Verification items for the finished model (mm, model axes). Coordinates: 2 decimals unless noted, no trailing zeros. Write each loop counter-clockwise with the first axis right and the second up, starting at its lowest first coordinate (ties: lowest second). Pieces come first, ordered by that corner, then holes. Notation, with made-up numbers: (-32.5, 65) - (13.5, 65) arc R21 ccw to (13.5, 86) - close; hole circle Ø6 at (38.25, 50). An arc over 180 degrees is marked (long way). Use one line per item in the form item = value. Start each with the question number.
(1) Gauge pin test, flat ends, axial feed: pin 1 Ø1 at (x, z) = (-4, -115) entering from -Y; pin 2 Ø5 at (y, z) = (-5, -49.5) entering from -X; pin 3 Ø6 at (y, z) = (-6, 46) entering from +X. Record the tip position at first contact, or that the pin passes through.
(2) Sectioned sample at B-B (y = 0). Record the cut outline in (x, z), and give its area (4 significant figures).
(3) Mould release check, pull along Y, two halves, no side actions. Record for faces 1 (the cylindrical face through (-1.713, -7.712, 2.275)), 2 (the flat face through (2, 6, 162.5)), 3 (the cylindrical face through (-1.301, -5.857, 2.275)): released by +Y, released by -Y, zero draft, split by the parting line, or undercut.
(4) Material ranges on line 1 (Z direction, x = 3, y = 5.75); line 2 (Y direction, x = 0, z = 89); line 3 (X direction, y = 2.75, z = -132.5), recorded low to high. Write a range as [from, to].
(5) Sectioned sample at C-C (z = -43.5). Record the cut outline in (x, y), and give its area (3 significant figures).
(6) Sectioned sample at A-A (x = 0). Record the cut outline in (y, z).
from build123d import *

# Parameters (mm, degrees)
CROQUIS1_R                 = 7.9
SALIENTE_EXTRUIR1_DEPTH    = 162.5
CROQUIS3_R                 = 6
CORTAR_EXTRUIR1_DEPTH      = 326.191974071
CORTAR_EXTRUIR2_REACH      = 164.884
CORTAR_EXTRUIR2_END_RADIUS = 7.9
CROQUIS4_W                 = 10
CROQUIS4_H                 = 10
CORTAR_EXTRUIR3_REACH      = 164.884
CORTAR_EXTRUIR3_END_RADIUS = 7.9
CROQUIS5_W                 = 9.290487028
CROQUIS5_H                 = 10


with BuildPart() as part:
    # Croquis1 → Saliente-Extruir1 (new, symmetric)
    with BuildSketch(Plane.XY):
        Circle(CROQUIS1_R)
    extrude(amount=SALIENTE_EXTRUIR1_DEPTH, both=True)

    # Croquis3 → Cortar-Extruir1 (cut, through all)
    with BuildSketch(Plane.XY.offset(162.5)):
        Circle(CROQUIS3_R)
    extrude(amount=-CORTAR_EXTRUIR1_DEPTH, mode=Mode.SUBTRACT)

    # Cortar-Extruir2: up to this cylinder (the profile starts inside it)
    cortar_extruir2_end = Plane(origin=(0, 0, 82.5), z_dir=(0, 0, -1)) * Cylinder(CORTAR_EXTRUIR2_END_RADIUS, 346.568, mode=Mode.PRIVATE)
    # Croquis4 → Cortar-Extruir2 (cut, up to the surface)
    with BuildSketch(Plane(origin=(0, 0, 0), x_dir=(1, 0, 0), z_dir=(0, 1, 0)), mode=Mode.PRIVATE) as cortar_extruir2_sk1:
        with Locations((0, -82.5)):
            Rectangle(CROQUIS4_W, CROQUIS4_H)
    cortar_extruir2_tool1 = extrude(cortar_extruir2_sk1.sketch, amount=CORTAR_EXTRUIR2_REACH, mode=Mode.PRIVATE) & cortar_extruir2_end
    add(cortar_extruir2_tool1.solids().sort_by_distance((0, 0, 82.5))[0], mode=Mode.SUBTRACT)

    # Cortar-Extruir3: up to this cylinder (the profile starts inside it)
    cortar_extruir3_end = Plane(origin=(0, 0, -67.5), z_dir=(0, 0, -1)) * Cylinder(CORTAR_EXTRUIR3_END_RADIUS, 346.568, mode=Mode.PRIVATE)
    # Croquis5 → Cortar-Extruir3 (cut, up to the surface)
    with BuildSketch(Plane(origin=(0, 0, 0), x_dir=(1, 0, 0), z_dir=(0, 1, 0)), mode=Mode.PRIVATE) as cortar_extruir3_sk1:
        with Locations((0, 67.5)):
            Rectangle(CROQUIS5_W, CROQUIS5_H)
    cortar_extruir3_tool1 = extrude(cortar_extruir3_sk1.sketch, amount=CORTAR_EXTRUIR3_REACH, mode=Mode.PRIVATE) & cortar_extruir3_end
    add(cortar_extruir3_tool1.solids().sort_by_distance((0, 0, -67.5))[0], mode=Mode.SUBTRACT)


solid = part.part
Answers below:
q1.pin_1 = -7.08
q1.pin_2 = -7.49
q1.pin_3 = 7.31
q2.outline = (-7.9, -162.5) - (-6, -162.5) - (-6, 162.5) - (-7.9, 162.5) - close; (6, -162.5) - (7.9, -162.5) - (7.9, 162.5) - (6, 162.5) - close
q2.area = 1,235 mm2
q3.face_1 = split by the parting line
q3.face_2 = zero draft
q3.face_3 = undercut
q4.line_1 = [-162.5, -72.5], [-62.5, 77.5], [87.5, 162.5]
q4.line_2 = [-7.9, -6], [6, 7.9]
q4.line_3 = [-7.41, -5.33], [5.33, 7.41]
q5.outline = circle Ø15.8 at (0, 0); hole circle Ø12 at (0, 0)
q5.area = 83.0 mm2
q6.outline = (-7.9, -162.5) - (-6, -162.5) - (-6, 162.5) - (-7.9, 162.5) - close; (6, -162.5) - (7.9, -162.5) - (7.9, -72.5) - (6, -72.5) - close; (6, -62.5) - (7.9, -62.5) - (7.9, 77.5) - (6, 77.5) - close; (6, 87.5) - (7.9, 87.5) - (7.9, 162.5) - (6, 162.5) - close
